Can you work these out from the drawing? Everything is in mm from the part's minimum corner. Round coordinates to 2 decimals unless told otherwise and drop trailing zeros. Loops run counter-clockwise (first coordinate to the right, second up) from the corner with the lowest first, then second, coordinate; pieces in that order, holes last. Notation, with made-up numbers: (62.25, 38) - (87.25, 38) arc R26 ccw to (87.25, 58) - close; hole circle Ø5 at (52, -14.75). An arc over 180 degrees is marked (long way). Answer as CSV lines item,"result". Start each with the question number.
1) Suppose I cut it at A-A, the plane y = 2.95. Write out the boundary of the cut face in (x, z).
2) Please list where these lines run through material, in increasing order: line 1 along X through (y, z) = (3.25, 45); line 2 along X through (y, z) = (2.5, 44.5) (1 decimal); line 3 along X through (y, z) = (3.6, 107).
3) Suppose I cut it at D-D, the plane x = 152. Write out the boundary of the cut face in (y, z), then the cut area to 3 significant figures.
4) Suppose I cut it at B-B, the plane z = 45. Write out the boundary of the cut face in (x, y).
5) Suppose I cut it at C-C, the plane z = 25. Write out the boundary of the cut face in (x, y) (1 decimal), then the cut area to 3 significant figures.
6) I'm going to push flat-ended pins straight in: pin 1 Ø2.5 at (y, z) = (1.5, 111.5) entering from -X; pin 2 Ø2.5 at (y, z) = (2.5, 107.5) entering from +X. Where does each tip first touch, or does it pass through?
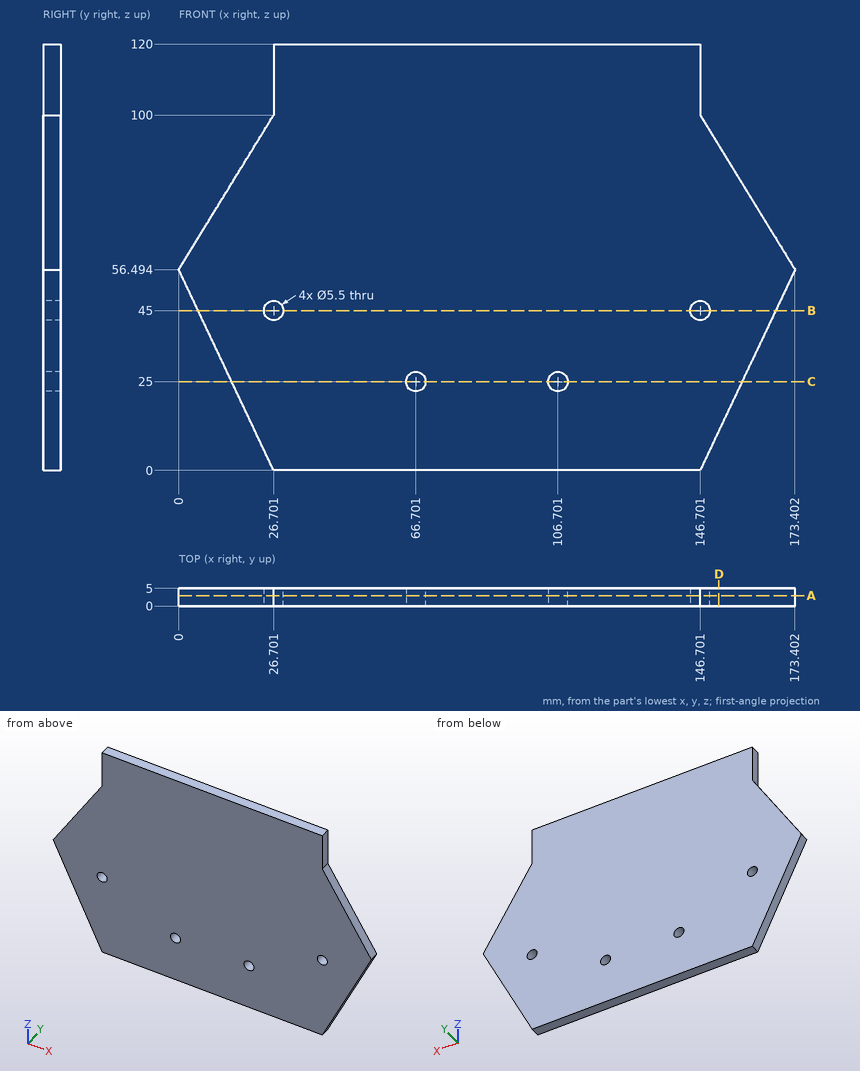
Filled sheet:
1,outline,"(0, 56.49) - (26.7, 0) - (146.7, 0) - (173.4, 56.49) - (146.7, 100) - (146.7, 120) - (26.7, 120) - (26.7, 100) - close; hole circle Ø5.5 at (26.7, 45); hole circle Ø5.5 at (66.7, 25); hole circle Ø5.5 at (106.7, 25); hole circle Ø5.5 at (146.7, 45)"
2,line 1,"5.43 to 23.95, 29.45 to 143.95, 149.45 to 167.97"
2,line 2,"5.7 to 24, 29.4 to 144, 149.4 to 167.7"
2,line 3,"26.7 to 146.7"
3,outline,"(0, 11.21) - (5, 11.21) - (5, 91.37) - (0, 91.37) - close"
3,area,"401 mm²"
4,outline,"(5.43, 0) - (23.95, 0) - (23.95, 5) - (5.43, 5) - close; (29.45, 0) - (143.95, 0) - (143.95, 5) - (29.45, 5) - close; (149.45, 0) - (167.97, 0) - (167.97, 5) - (149.45, 5) - close"
5,outline,"(14.9, 0) - (64, 0) - (64, 5) - (14.9, 5) - close; (69.5, 0) - (104, 0) - (104, 5) - (69.5, 5) - close; (109.5, 0) - (158.5, 0) - (158.5, 5) - (109.5, 5) - close"
5,area,"663 mm²"
6,pin 1,"x = 26.7"
6,pin 2,"x = 146.7"
